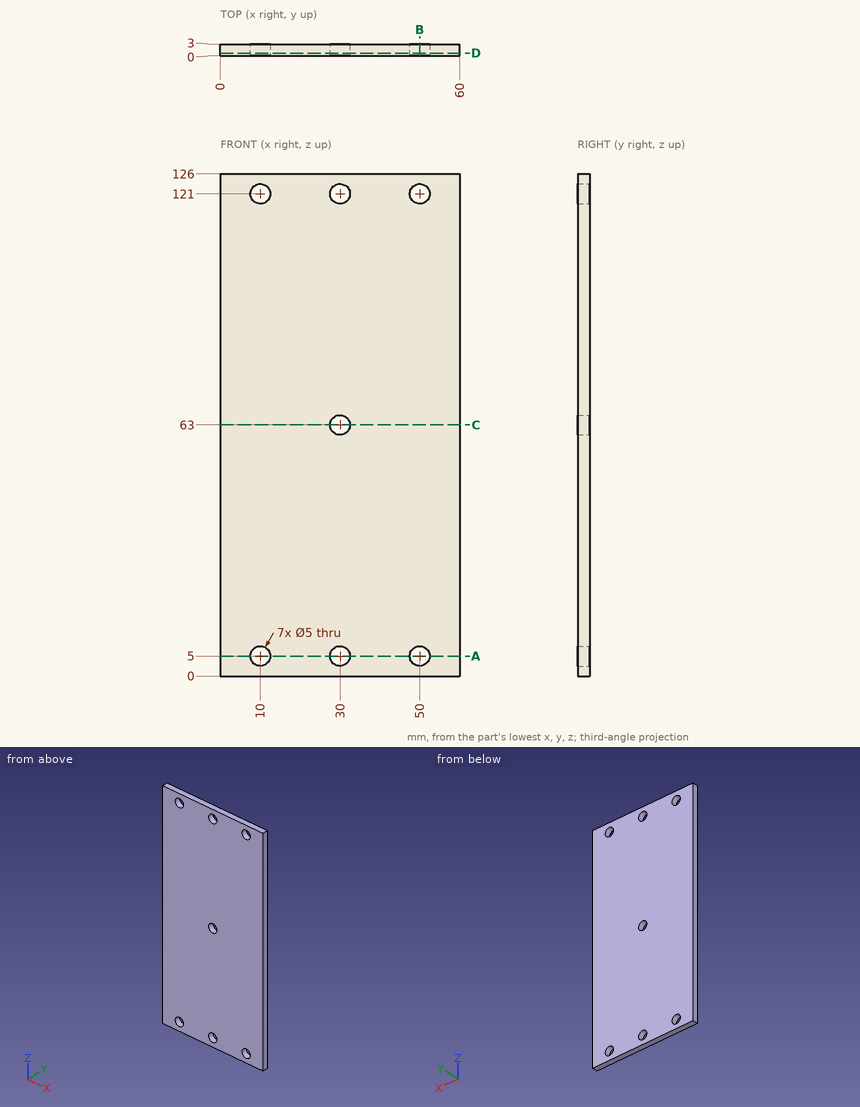
Can you work these out from the drawing? Everything is in mm from the part's minimum corner. Round coordinates to 2 decimals unless told otherwise and drop trailing zeros. Loops run counter-clockwise (first coordinate to the right, second up) from the corner with the lowest first, then second, coordinate; pieces in that order, holes last. Notation, with made-up numbers: (19, -22) -> (52, -22) arc R9 cw to (52, -7) -> close; hole circle Ø8 at (58.5, 11.25). An arc over 180 degrees is marked (long way). Put each result on its own line as item: value.
Q1. Please list where these lines run through material, in increasing order: line 1 (Z direction, x = 30, y = 1.15); line 2 (Z direction, x = 50, y = 1); line 3 (X direction, y = 1.95, z = 121). Write a range as from..to.
Checks:
line 1: 0..2.5, 7.5..60.5, 65.5..118.5, 123.5..126
line 2: 0..2.5, 7.5..118.5, 123.5..126
line 3: 0..7.5, 12.5..27.5, 32.5..47.5, 52.5..60
Q2. I want a section at B-B on x = 50. Write out the boundary of the cut face in (y, z).
Checks:
outline: (0, 0) -> (3, 0) -> (3, 2.5) -> (0, 2.5) -> close; (0, 7.5) -> (3, 7.5) -> (3, 118.5) -> (0, 118.5) -> close; (0, 123.5) -> (3, 123.5) -> (3, 126) -> (0, 126) -> close
Q3. I want a section at C-C on z = 63. Write out the boundary of the cut face in (x, y).
Checks:
outline: (0, 0) -> (27.5, 0) -> (27.5, 3) -> (0, 3) -> close; (32.5, 0) -> (60, 0) -> (60, 3) -> (32.5, 3) -> close
Q4. I want a section at A-A on z = 5. Write out the boundary of the cut face in (x, y), and give its area (3 significant figures).
Checks:
outline: (0, 0) -> (7.5, 0) -> (7.5, 3) -> (0, 3) -> close; (12.5, 0) -> (27.5, 0) -> (27.5, 3) -> (12.5, 3) -> close; (32.5, 0) -> (47.5, 0) -> (47.5, 3) -> (32.5, 3) -> close; (52.5, 0) -> (60, 0) -> (60, 3) -> (52.5, 3) -> close
area: 135 mm2
Q5. For pin 1 Ø6 at (x, z) = (10, 5) entering from +Y, with a flat end and sliding along its axis, tell me the tip position at first contact or that it passes through.
Checks:
pin 1: y = 3
Q6. I want a section at D-D on y = 0.7. Write out the boundary of the cut face in (x, z).
Checks:
outline: (0, 0) -> (60, 0) -> (60, 126) -> (0, 126) -> close; hole circle Ø5 at (10, 5); hole circle Ø5 at (10, 121); hole circle Ø5 at (30, 5); hole circle Ø5 at (30, 63); hole circle Ø5 at (30, 121); hole circle Ø5 at (50, 5); hole circle Ø5 at (50, 121)
